```python
from build123d import *

# Parameters (mm, degrees)
EXTRUDE_1_DEPTH     = 17
CUT_EXTRUDE_1_DEPTH = 10


with BuildPart() as part:
    # 草圖1 → 填料-伸長1 (new body)
    with BuildSketch(Plane(origin=(0, 0, 0), x_dir=(1, 0, 0), z_dir=(0, 1, 0))):
        with BuildLine():
            Line((28, 26), (36, 26))
            ThreePointArc((36, 26), (39.535533906, 24.535533906), (41, 21))
            Line((41, 21), (41, -21))
            ThreePointArc((41, -21), (39.535533906, -24.535533906), (36, -26))
            Line((36, -26), (28, -26))
            Line((28, -26), (20, -22.5))
            Line((20, -22.5), (-20, -22.5))
            Line((-20, -22.5), (-28, -26))
            Line((-28, -26), (-36, -26))
            ThreePointArc((-36, -26), (-39.535533906, -24.535533906), (-41, -21))
            Line((-41, -21), (-41, 21))
            ThreePointArc((-41, 21), (-39.535533906, 24.535533906), (-36, 26))
            Line((-36, 26), (-28, 26))
            Line((-28, 26), (-20, 22.5))
            Line((-20, 22.5), (20, 22.5))
            Line((20, 22.5), (28, 26))
        make_face()
    extrude(amount=EXTRUDE_1_DEPTH)

    # 草圖2 → 除料-伸長1 (cut)
    with BuildSketch(Plane(origin=(0, 0, -22.5), x_dir=(-1, 0, 0), z_dir=(0, 0, -1))):
        with BuildLine():
            Line((14.85, 6.6), (10.15, 6.6))
            ThreePointArc((10.15, 6.6), (8.25, 8.5), (10.15, 10.4))
            Line((10.15, 10.4), (14.85, 10.4))
            ThreePointArc((14.85, 10.4), (16.75, 8.5), (14.85, 6.6))
        make_face()
    extrude(amount=-CUT_EXTRUDE_1_DEPTH, mode=Mode.SUBTRACT)


solid = part.part
```
Can you work these out from the model? Positions are in its coordinate system, mm. A direction names the side the tool comes from. Coordinates: 2 decimals unless noted, no trailing zeros. Loops run counter-clockwise (first coordinate to the right, second up) from the corner with the lowest first, then second, coordinate; pieces in that order, holes last. Notation, with made-up numbers: M 38,-6 L 85,-6 A23 ccw 85,18 Z; hole C -14.75,53.25 d5. An arc over 180 degrees is marked long. Put each result on its own line as item: value. Start each with the question number.
(1) We'd pull the mould along X, two halves only. Please class faces 1 (the face through (-39, 8, 25)), 2 (the face through (23.944, 8.381, -24.226)), 3 (the face through (1, 0, 0)), 4 (the face through (39, 8, -25)): +X half, -X half, draft (parallel to the pull), parting line (faces both ways), or undercut.
(2) Imagine slicing it at B-B on x = 15. List the corners of the cut face in (y, z) for me.
(3) I need wall thicknesses on probe 1 along Z at (x, y) = (-9.5, 16); probe 2 along Z at (x, y) = (-27, 16); probe 3 along X at (y, z) = (9.25, -13.5). Which ranges of each line are inside material? Lowest first, please.
(4) Imagine slicing it at D-D on x = -23.5. List the corners of the cut face in (y, z) for me, and give its area (3 significant figures).
(5) Imagine slicing it at A-A on y = 8.5. List the corners of the cut face in (x, z) for me, and give its area (3 significant figures).
(6) Imagine slicing it at C-C on y = 4.5. List the corners of the cut face in (x, z) for me, and give its area (3 significant figures).
(7) Which directions (+Z, -Z, +X, -X, +Y, -Y) give clear straight access to the entire face, cutting with the end or side of a thin tool? Please do faces 5 (the face through (-23.944, 8.381, 24.226)), 6 (the face through (32, 8, 26)), 7 (the face through (-24.056, 8.381, -24.274)), 8 (the face through (1, 17, 0)), 9 (the face through (-13, 6.6, -18)).
(8) Will these pins go through, and if not, where does the flat tip stop? pin 1 Ø4 at (x, z) = (-13, -16.5) entering from -Y; pin 2 Ø4 at (x, y) = (-14, 8.5) entering from -Z; pin 3 Ø1.5 at (x, y) = (6.5, 3) entering from +Z.
Worked answers:
1. face 1: -X half
1. face 2: undercut
1. face 3: draft
1. face 4: +X half
2. outline: M 0,-22.5 L 17,-22.5 L 17,22.5 L 0,22.5 Z
3. probe 1: z = -22.5 to 22.5
3. probe 2: z = -25.56 to 25.56
3. probe 3: x = -41 to -16.6, -8.4 to 41
4. outline: M 0,-24.03 L 17,-24.03 L 17,24.03 L 0,24.03 Z
4. area: 817 mm2
5. outline: M -41,-21 A5 ccw -36,-26 L -28,-26 L -20,-22.5 L -16.75,-22.5 L -16.75,-12.5 L -8.25,-12.5 L -8.25,-22.5 L 20,-22.5 L 28,-26 L 36,-26 A5 ccw 41,-21 L 41,21 A5 ccw 36,26 L 28,26 L 20,22.5 L -20,22.5 L -28,26 L -36,26 A5 ccw -41,21 Z
5. area: 3,820 mm2
6. outline: M -41,-21 A5 ccw -36,-26 L -28,-26 L -20,-22.5 L 20,-22.5 L 28,-26 L 36,-26 A5 ccw 41,-21 L 41,21 A5 ccw 36,26 L 28,26 L 20,22.5 L -20,22.5 L -28,26 L -36,26 A5 ccw -41,21 Z
6. area: 3,910 mm2
7. face 5: +Z, +Y, -Y
7. face 6: +Z, +X, -X, +Y, -Y
7. face 7: -Z, +Y, -Y
7. face 8: +Z, -Z, +X, -X, +Y
7. face 9: -Z
8. pin 1: stops at y = 0
8. pin 2: stops at z = -22.5
8. pin 3: stops at z = 22.5
